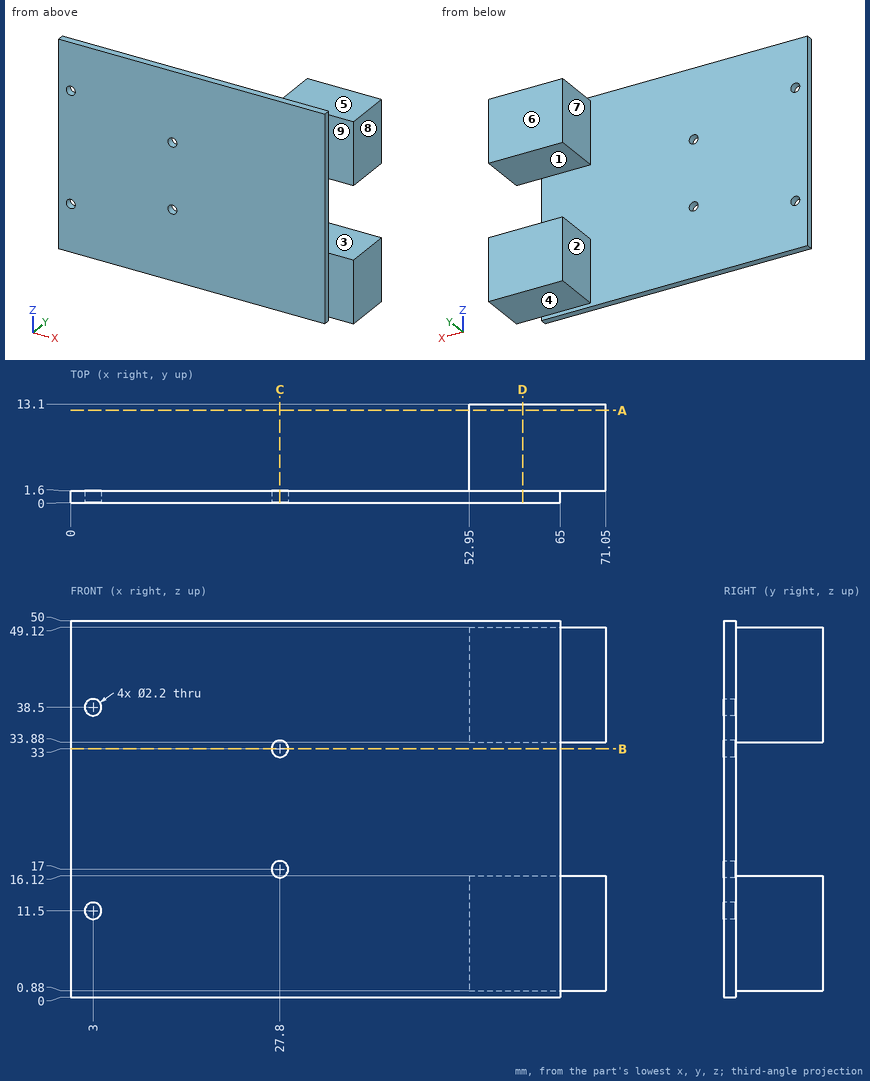
Geometry: see drawing. Coordinates: mm, zero at the bounding-box minimum. A direction names the side the tool comes from. Coordinates: 2 decimals unless noted, no trailing zeros. Order: outer loops, then holes, each group sorted by start corner. A loop starts at its lowest first (then second) coordinate and runs counter-clockwise, first axis right, second up. Notation, with made-up numbers: M -34,-21.75 L 17,-21.75 A4 cw 17,-15.75 Z; hole C 63,67.5 d11. An arc over 180 degrees is marked long. Write item = value, one per line. Start each with the question number.
(1) Section D-D on x = 60. Output: boundary loops of the cut face in (y, z).
(2) Section C-C on x = 27.8. Output: boundary loops of the cut face in (y, z).
(3) First-contact query: P1, Ø6, axis at y = 8, z = 8, coming from the -X side; P2, Ø2.5, axis at x = 27.8, z = 17, coming from the +Y side; P3, Ø2, axis at x = 27.8, z = 33, coming from the +Y side; P4, Ø3, axis at x = 68.5, z = 45, coming from the -Y side. Flat tips, straight axial feed; report the tip coordinate or a pass-through.
(4) Section A-A on y = 12.25. Output: boundary loops of the cut face in (x, z).
(5) Pull-direction query (Z, two-part tool) for the marked faces 1, 2, 3 and 4; classes: released by +Z, released by -Z, zero draft, split by the parting line, or undercut.
(6) Line query: line 1 along Z through (x, y) = (3, 0.75); line 2 along X through (y, z) = (0.55, 38.5); line 3 along Z through (x, y) = (63, 6.5). Output: solid intervals per line, ascending. Write a range as [from, to].
(7) Section B-B on z = 33. Output: boundary loops of the cut face in (x, y).
(8) Reachability of the marked faces 5, 6, 7, 8 and 9 from +Z, -Z, +X, -X, +Y, -Y: full face, straight path, thin tool, end or side. Return the list, or none.
Result set:
q1.outline = M 0,0 L 1.6,0 L 1.6,0.88 L 13.1,0.88 L 13.1,16.12 L 1.6,16.12 L 1.6,33.88 L 13.1,33.88 L 13.1,49.12 L 1.6,49.12 L 1.6,50 L 0,50 Z
q2.outline = M 0,0 L 1.6,0 L 1.6,15.9 L 0,15.9 Z; M 0,18.1 L 1.6,18.1 L 1.6,31.9 L 0,31.9 Z; M 0,34.1 L 1.6,34.1 L 1.6,50 L 0,50 Z
q3.P1 = 52.95
q3.P2 = 1.6
q3.P3 = through
q3.P4 = 1.6
q4.outline = M 52.95,0.88 L 71.05,0.88 L 71.05,16.12 L 52.95,16.12 Z; M 52.95,33.88 L 71.05,33.88 L 71.05,49.12 L 52.95,49.12 Z
q5.face_1 = undercut
q5.face_2 = zero draft
q5.face_3 = undercut
q5.face_4 = released by -Z
q6.line_1 = [0, 10.4], [12.6, 37.4], [39.6, 50]
q6.line_2 = [0, 1.9], [4.1, 65]
q6.line_3 = [0.88, 16.12], [33.88, 49.12]
q7.outline = M 0,0 L 26.7,0 L 26.7,1.6 L 0,1.6 Z; M 28.9,0 L 65,0 L 65,1.6 L 28.9,1.6 Z
q8.face_5 = +Z, +X, -X, +Y
q8.face_6 = +Z, -Z, +X, -X, +Y
q8.face_7 = +Z, -Z, -X, +Y
q8.face_8 = +Z, -Z, +X, +Y, -Y
q8.face_9 = +Z, -Z, +X, -Y
